from build123d import *

# Parameters (mm, degrees)
SKETCH_1_W          = 17
SKETCH_1_H          = 23
EXTRUDE_1_DEPTH     = 8.5
CUT_EXTRUDE_1_DEPTH = 20
SKETCH_3_W          = 15
SKETCH_3_H          = 21
EXTRUDE_2_DEPTH     = 3.5
SKETCH_4_R          = 8.5
EXTRUDE_3_DEPTH     = 6.5
SKETCH_5_R          = 7
EXTRUDE_4_DEPTH     = 22
SKETCH_6_W          = 3
SKETCH_6_H          = 0.5
EXTRUDE_5_DEPTH     = 8
SKETCH_7_R          = 6.5
EXTRUDE_6_DEPTH     = 0.01


with BuildPart() as part:
    # ｽｹｯﾁ1 → ﾎﾞｽ - 押し出し1 (new body)
    with BuildSketch(Plane.XY):
        Rectangle(SKETCH_1_W, SKETCH_1_H)
    extrude(amount=EXTRUDE_1_DEPTH)

    # ｽｹｯﾁ2 → ｶｯﾄ - 押し出し1 (cut)
    with BuildSketch(Plane(origin=(8.5, 0, 0), x_dir=(0, 0, -1), z_dir=(1, 0, 0))):
        Polygon((-8.5, 11), (-7, 11), (-5, 9), (-5, -9), (-7, -11), (-8.5, -11), align=None)
    extrude(amount=-CUT_EXTRUDE_1_DEPTH, mode=Mode.SUBTRACT)

    # ｽｹｯﾁ3 → ﾎﾞｽ - 押し出し2 (add)
    with BuildSketch(Plane.XY.offset(5)):
        Rectangle(SKETCH_3_W, SKETCH_3_H)
    extrude(amount=EXTRUDE_2_DEPTH)

    # ｽｹｯﾁ4 → ﾎﾞｽ - 押し出し3 (add)
    with BuildSketch(Plane(origin=(0, 0, 0), x_dir=(-1, 0, 0), z_dir=(0, 0, -1))):
        Circle(SKETCH_4_R)
    extrude(amount=EXTRUDE_3_DEPTH)

    # ｽｹｯﾁ5 → ﾎﾞｽ - 押し出し4 (add)
    with BuildSketch(Plane(origin=(0, 0, 0), x_dir=(-1, 0, 0), z_dir=(0, 0, -1))):
        Circle(SKETCH_5_R)
    extrude(amount=EXTRUDE_4_DEPTH)

    # ｽｹｯﾁ6 → ﾎﾞｽ - 押し出し5 (add)
    with BuildSketch(Plane(origin=(0, 0, -22), x_dir=(-1, 0, 0), z_dir=(0, 0, -1))):
        with Locations((-4.266281297, 2.75)):
            Rectangle(SKETCH_6_W, SKETCH_6_H)
        with Locations((0, 2.75)):
            Rectangle(SKETCH_6_W, SKETCH_6_H)
        with Locations((4.5, 2.75)):
            Rectangle(SKETCH_6_W, SKETCH_6_H)
    extrude(amount=EXTRUDE_5_DEPTH)

    # ｽｹｯﾁ7 → ﾎﾞｽ - 押し出し6 (add)
    with BuildSketch(Plane(origin=(0, 0, -22), x_dir=(-1, 0, 0), z_dir=(0, 0, -1))):
        Circle(SKETCH_7_R)
    extrude(amount=EXTRUDE_6_DEPTH)


solid = part.part
Geometry check sheet. Reference: the model listing, model coordinates, mm. A direction names the side the tool comes from. Round coordinates to 2 decimals unless told otherwise and drop trailing zeros. Write each loop counter-clockwise with the first axis right and the second up, starting at its lowest first coordinate (ties: lowest second). Pieces come first, ordered by that corner, then holes. Notation, with made-up numbers: (11.25, 52) -> (67.25, 52) arc R21 cw to (67.25, 71) -> close; hole circle Ø9 at (-18.5, -7). An arc over 180 degrees is marked (long way). One line per item, written item: value. Start each with the question number.
(1) Access from +Z, -Z, +X, -X, +Y, -Y to the whole of each face (thin tool, end or side, straight path). Record for faces 5 (the cylindrical face through (-4.57, 7.167, -3.204)), 6 (the flat face through (4, 3, -26)), 7 (the flat face through (0, 10, 0)), 8 (the flat face through (0, 11, 8)), 9 (the flat face through (-7.5, 0, 7)).
(2) Cross-section at B-B, the plane z = -17.5. Record the cut outline in (x, y).
(3) Draft check along Y on faces 1 (the flat face through (-8.5, 0, 2)), 2 (the flat face through (0, -10.7, 6.7)), 3 (the flat face through (0, 11.5, 4)), 4 (the flat face through (8, 0, 5)). Enter one of: +Y half, -Y half, draft (parallel to the pull), parting line (faces both ways), or undercut.
(4) Scan lines: line 1 (Y direction, x = 4.25, z = -25.5); line 2 (Z direction, x = 2, y = -1); line 3 (Z direction, x = -7.25, y = -5.25). Record each from-to range of solid material in increasing order. Write a range as [from, to].
(5) Go/stop test with flat-tipped pins: pin 1 Ø8 at (x, z) = (-6.5, -23) entering from -Y; pin 2 Ø6 at (x, y) = (-3, -5.5) entering from -Z; pin 3 Ø10 at (y, z) = (1.5, -23) entering from +X. Record where each tip stops, or that it passes through.
Answer:
1. face 5: -Z
1. face 6: -Z, +X, -X, +Y
1. face 7: -Z, +Y
1. face 8: +Z, +X, -X
1. face 9: +Z, -X
2. outline: circle Ø14 at (0, 0)
3. face 1: draft
3. face 2: undercut
3. face 3: +Y half
3. face 4: undercut
4. line 1: [2.5, 3]
4. line 2: [-22.01, 8.5]
4. line 3: [0, 8.5]
5. pin 1: y = -6.49
5. pin 2: z = -22.01
5. pin 3: x = 7
